Autodesk Inventor part; units mm, degrees
ref_plane "Work Plane1" through (29, 0, 0) normal (0, -1, 0) x (1, 0, 0)
ref_plane "YZ Plane" through (0, 0, 0) normal (1, 0, 0) x (0, 1, 0)
ref_plane "XZ Plane" through (0, 0, 0) normal (0, 1, 0) x (-1, 0, 0)
sketch "Szkic1" plane through (0, 0, 0) normal (0, 0, 1) x (1, 0, 0)
  line L0 (-0.7333, 0) -> (20, 0)
  line L1 (20, 0) -> (20, 1.25)
  line L2 (20, 1.25) -> (1.125, 1.25)
  line L3 (1.125, 1.25) -> (0.8488, 1.25)
  line L4 (0.8488, 1.25) -> (0, 1.25)
  line L5 (0, 1.25) -> (0, 2.25)
  line L6 (0, 2.25) -> (-2.5, 2.25)
  line L7 (-2.5, 2.25) -> (-2.5, 1.1547)
  line L8 (-2.5, 1.1547) -> (-1.4, 1.1547)
  line L9 (-1.4, 1.1547) -> (-0.7333, 0)
  line L10 (-7, 0) -> (24.5, 0)
  line L11 (0, -0.45) -> (0, 2.7)
  line L12 (1.125, 1.25) -> (0, 1.25) construction
  dimension "d1" = 18.875
  dimension "d2" = 0.2762
  dimension "d3" = 2.5
  dimension "d4" = 1.1
  dimension "d5" = 60
  dimension "d6" = 2.5
  dimension "d7" = 2.5
  dimension "d8" = 2.3094
  dimension "d9" = 4.5
  dimension "d26" = 20
revolve "Bryła" add sketch "Szkic1" angle 360 about axis through (-0.7333, 0, 0) along (1, 0, 0)
sketch "Szkic2" plane through (-2.5, 0, 0) normal (-1, 0, 0) x (0, 0, 1)
  circle A0 centre (0, 0) radius 1.1547
  line L0 (0, -3.15) -> (0, 3.15)
  line L1 (-3.15, 0) -> (3.15, 0)
  line L2 (1.1547, 0) -> (0.5774, -1)
  line L3 (0.5774, -1) -> (-0.5774, -1)
  line L4 (-0.5774, -1) -> (-1.1547, 0)
  line L5 (-1.1547, 0) -> (-0.5774, 1)
  line L6 (-0.5774, 1) -> (0.5774, 1)
  line L7 (0.5774, 1) -> (1.1547, 0)
extrude "Szczelina" add sketch "Szkic2" against normal up to next contours L7 A0 | A0 L2 | L6 L0 A0 | A0 L0 L3 | L0 L6 A0 | A0 L3 L0 | L4 A0 | A0 L5
fillet "Zaokrąglenie1" radius 0.25 1 edges at (-2.5, -2.25, 0)
thread "Gwint"
chamfer "Faza1" distance 0.2761 distance2 0.2761 1 edges at (20, -1.25, 0) measured on face at (20, -0.2763, -0.017)
ref_plane "Work Plane1" through (29, 0, 0) normal (0, -1, 0) x (1, 0, 0)
fillet "Fillet2" radius 0.1 1 edges at (0, -1.25, 0)
equation "\"d1\" = GEL"
equation "\"d3\" = KOH"
equation "\"d4\" = INTI"
equation "\"d6\" = GD"
equation "\"d7\" = BDM"
equation "\"d8\" = 1.1547 * SW"
equation "\"d9\" = KOD"
equation "\"d26\" = NLG"
equation "\"d30\" = R"
equation "\"d17\" = RR"
equation "\"d13\" = GEL"
equation "\"d15\" = -0.5 * SPD + 0.5 * GD"
equation "\"d16\" = GUL"
equation "\"GD\" = NND"
equation "\"NLG\" = 20"
equation "\"GEL\" = 18.875"
equation "\"KOD\" = 4.5"
equation "\"KOH\" = 2.5"
equation "\"INTI\" = 1.1"
equation "\"GAL\" = 0.61345 * PTC"
equation "\"GUL\" = 0.61345 * PTC"
equation "\"BDM\" = NND"
equation "\"SW\" = 2"
equation "\"RR\" = 0.25"
equation "\"SPD\" = NND - 1.2269 * PTC"
equation "\"R\" = 0.1"
equation "\"TOA\" = 30deg"
equation "\"GD1\" = THREADDIA - 1.2269 * PTC"
equation "\"THREADDIA\" = 2.5"
equation "\"FAWI\" = 45deg"
equation "\"ANG\" = 120deg"
equation "\"PTC\" = 0.45"
equation "\"NND\" = 2.5"
equation "\"E0\" = 1.155 * SW"
properties part number "DIN 912 - M2,5 x 20" material "Stal, miękka"
Source: CAD feature listing. Evaluate the final solid. Frame: model axes, mm. A direction names the side the tool comes from. Round coordinates to 2 decimals unless told otherwise and drop trailing zeros. Loops run counter-clockwise (first coordinate to the right, second up) from the corner with the lowest first, then second, coordinate; pieces in that order, holes last. Notation, with made-up numbers: (14.5, -37) - (35.5, -37) arc R29 ccw to (35.5, -11) - close; hole circle Ø1 at (-12, -9.75). An arc over 180 degrees is marked (long way). Write item = value, one per line. Start each with the question number.
(1) Set-up query: faces 4 (the face through (-1.91, -0.51, -0.86)), 5 (the face through (0, 0.5, -1.5)), 6 (the face through (-2.5, -1, 1)). Return all of +Z, -Z, +X, -X, +Y, -Y with unobstructed straight access to the full face (end or side cutting, diameter ignored); none if empty.
(2) Pin query (flat end, axial travel): pin 1 (1.5 mm diameter, centred on x = 17.5, z = -1, fed in from -Y). Return the tip coordinate at first contact, or that it passes through.
(3) Pull-direction query (Z, two-part tool) for faces 1 (the face through (20, 0, 0)), 2 (the face through (9.77, -0.27, 1.22)), 3 (the face through (-1.91, -0.49, 0.87)); classes: +Z half, -Z half, draft (parallel to the pull), parting line (faces both ways), or undercut.
(4) Ray query, line 1 along X through (y, z) = (1.55, -1.05); line 2 along Z through (x, y) = (-0.25, -0.8); line 3 along X through (y, z) = (-0.3, 0.75). Return the intervals inside material, ascending. Write a range as from..to.
(5) Section query A-A, the plane x = 5.5. Output: boundary loops of the cut face in (y, z).
Conclusion:
q1.face_4 = -X
q1.face_5 = +X
q1.face_6 = +Z, -Z, -X, +Y, -Y
q2.pin_1 = -1.22
q3.face_1 = draft
q3.face_2 = parting line
q3.face_3 = undercut
q4.line_1 = -2.5..0
q4.line_2 = -2.1..2.1
q4.line_3 = -1.2..20
q5.outline = circle Ø2.5 at (0, 0)
